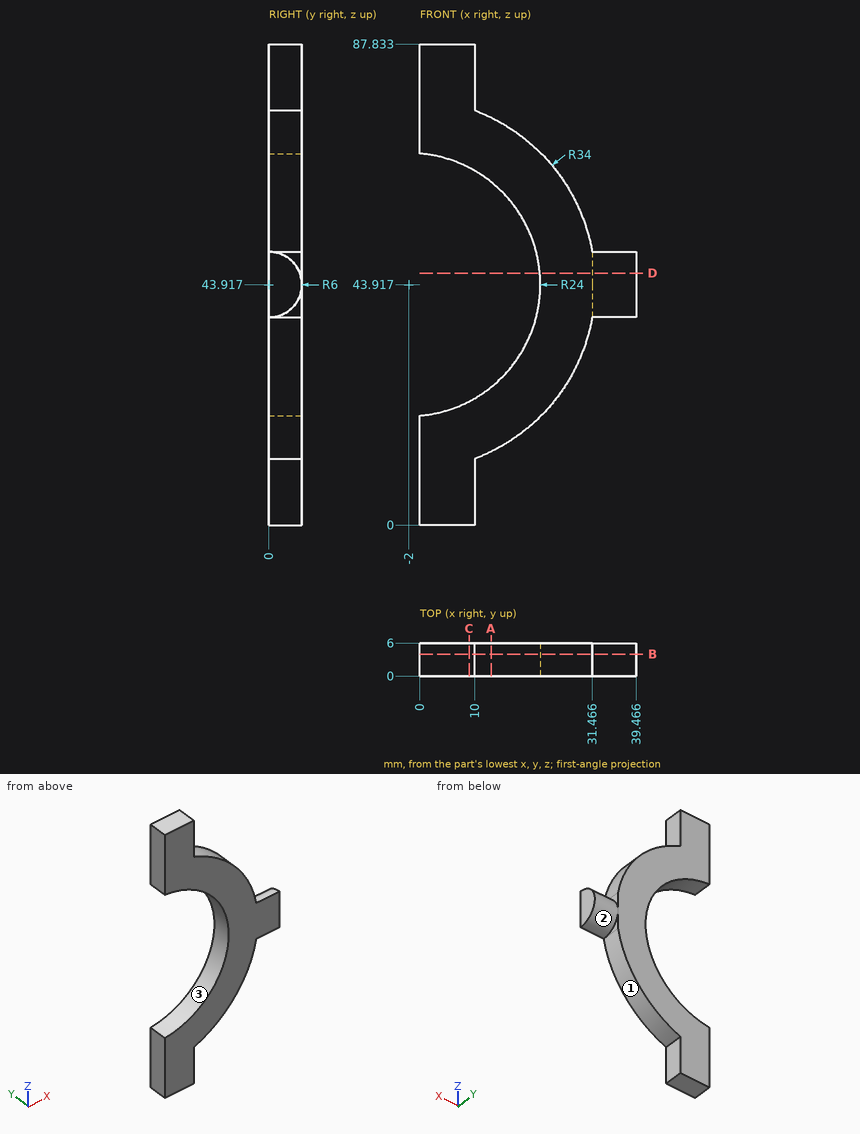
Can you work these out from the drawing? Everything is in mm from the part's minimum corner. Give positions to 0.01 mm unless a question says otherwise; leave off trailing zeros. Loops run counter-clockwise (first coordinate to the right, second up) from the corner with the lowest first, then second, coordinate; pieces in that order, holes last. Notation, with made-up numbers: (-19.75, 46) -> (-11.75, 46) arc R19 cw to (-11.75, 55) -> close; hole circle Ø1 at (11, 15.25). An arc over 180 degrees is marked (long way). Put each result on its own line as item: value.
(1) Please list where these lines run through material, in increasing order: probe 1 along X at (y, z) = (4, 12); probe 2 along Z at (x, y) = (7, 2.95) (1 decimal); probe 3 along Z at (x, y) = (14.5, 2.25) (1 decimal). Write a range as [from, to].
Computed:
probe 1: [0, 10]
probe 2: [0, 21.7], [66.2, 87.8]
probe 3: [14.2, 26.5], [61.3, 73.6]
(2) Imagine slicing it at B-B on y = 4. Write out the boundary of the cut face in (x, z) (1 decimal), plus the area to 3 significant figures.
Computed:
outline: (0, 0) -> (10, 0) -> (10, 12.1) arc R34 ccw to (31.5, 37.9) -> (31.5, 39.4) -> (39.5, 39.4) -> (39.5, 48.4) -> (31.5, 48.4) -> (31.5, 49.9) arc R34 ccw to (10, 75.7) -> (10, 87.8) -> (0, 87.8) -> (0, 67.8) arc R24 cw to (0, 20) -> close
area: 1,150 mm^2
(3) Imagine slicing it at A-A on x = 13. Write out the boundary of the cut face in (y, z) (1 decimal).
Computed:
outline: (0, 13.4) -> (6, 13.4) -> (6, 25.2) -> (0, 25.2) -> close; (0, 62.7) -> (6, 62.7) -> (6, 74.4) -> (0, 74.4) -> close
(4) Imagine slicing it at C-C on x = 9. Write out the boundary of the cut face in (y, z) (1 decimal), plus the area to 3 significant figures.
Computed:
outline: (0, 0) -> (6, 0) -> (6, 22.6) -> (0, 22.6) -> close; (0, 65.2) -> (6, 65.2) -> (6, 87.8) -> (0, 87.8) -> close
area: 271 mm^2
(5) I'm going to push flat-ended pins straight in: pin 1 Ø1 at (x, y) = (34.5, 2.5) entering from +Z; pin 2 Ø3 at (x, y) = (12.5, 4) entering from -Z; pin 3 Ø3 at (y, z) = (4.5, 6.5) entering from +X; pin 4 Ø1.5 at (y, z) = (3.5, 11) entering from -X. Where does each tip first touch, or does it pass through?
Computed:
pin 1: z = 49.57
pin 2: z = 12.5
pin 3: x = 10
pin 4: x = 0
(6) Imagine slicing it at D-D on z = 46. Write out the boundary of the cut face in (x, y).
Computed:
outline: (21.91, 0) -> (39.47, 0) -> (39.47, 5.63) -> (31.47, 5.63) -> (31.47, 6) -> (21.91, 6) -> close
(7) Thinking about a two-plate mould opening in Z: for the marked faces 1, 2 and 3, which applies, pulls with the +Z half, pulls with the -Z half, needs draft (parallel to the pull), parting line crosses it, or undercut?
Computed:
face 1: pulls with the -Z half
face 2: parting line crosses it
face 3: undercut
